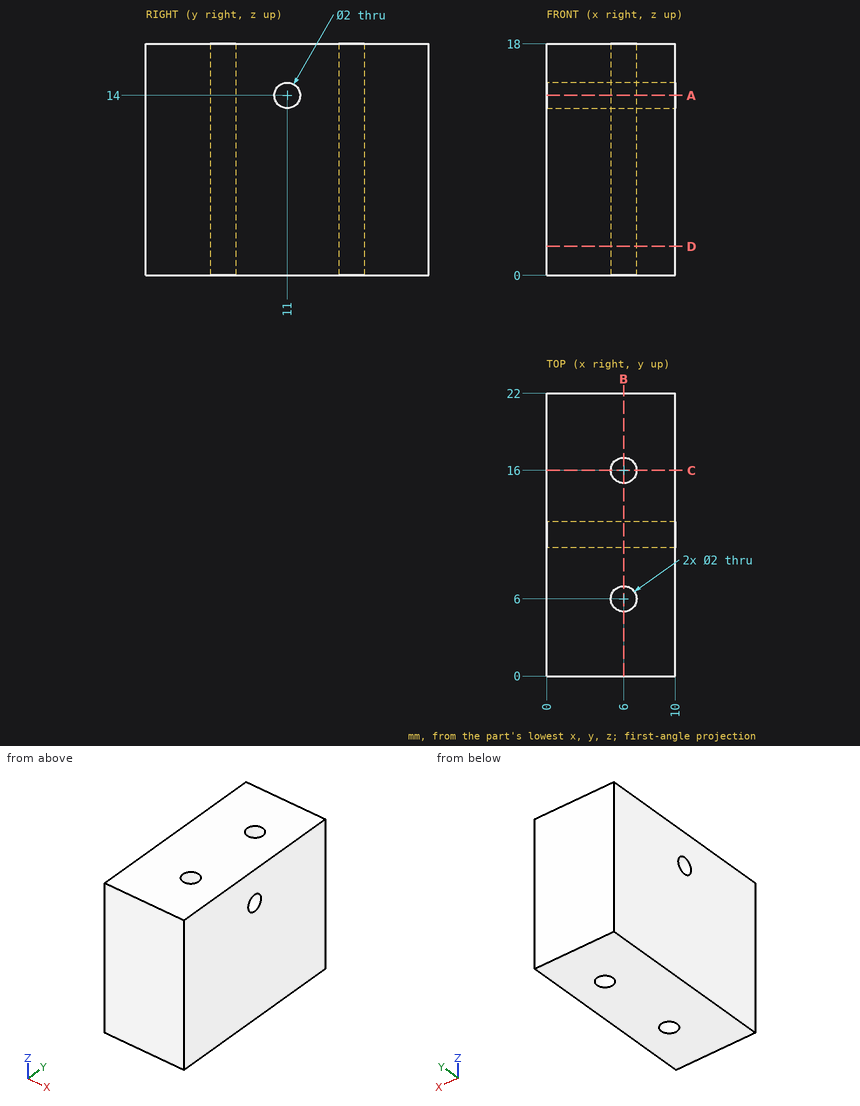
Input: dimensioned drawing with shaded views. Units: mm. Origin: part minimum x, y, z. Give positions to 0.01 mm unless a question says otherwise; leave off trailing zeros. Order: outer loops, then holes, each group sorted by start corner. A loop starts at its lowest first (then second) coordinate and runs counter-clockwise, first axis right, second up. Notation, with made-up numbers: (-33.5, -2.5) -> (-27.5, -2.5) arc R20 ccw to (-27.5, 21.5) -> close; hole circle Ø7 at (-19, -39.5). An arc over 180 degrees is marked (long way). Write item = value, one per line.
Item 1: Section query B-B (x = 6). Output: boundary loops of the cut face in (y, z), then the cut area to 3 significant figures.
Check result:
outline = (0, 0) -> (5, 0) -> (5, 18) -> (0, 18) -> close; (7, 0) -> (15, 0) -> (15, 18) -> (7, 18) -> close; (17, 0) -> (22, 0) -> (22, 18) -> (17, 18) -> close; hole circle Ø2 at (11, 14)
area = 321 mm²
Item 2: Ray query, probe 1 along Y at (x, z) = (6, 12); probe 2 along X at (y, z) = (6, 8); probe 3 along X at (y, z) = (6.5, 3). Return the intervals inside material, ascending.
Check result:
probe_1 = 0 to 5, 7 to 15, 17 to 22
probe_2 = 0 to 5, 7 to 10
probe_3 = 0 to 5.13, 6.87 to 10
Item 3: Section query C-C (y = 16). Output: boundary loops of the cut face in (x, z), then the cut area to 3 significant figures.
Check result:
outline = (0, 0) -> (5, 0) -> (5, 18) -> (0, 18) -> close; (7, 0) -> (10, 0) -> (10, 18) -> (7, 18) -> close
area = 144 mm²
Item 4: Contact query for a flat-ended pin moving along its axis: pin 1 (1.6 mm diameter, centred on x = 6, y = 16, fed in from -Z) (3 decimals). Output: stop coordinate, or through.
Check result:
pin_1 = through
Item 5: Section query A-A (z = 14). Output: boundary loops of the cut face in (x, y).
Check result:
outline = (0, 0) -> (10, 0) -> (10, 10) -> (0, 10) -> close; (0, 12) -> (10, 12) -> (10, 22) -> (0, 22) -> close; hole circle Ø2 at (6, 6); hole circle Ø2 at (6, 16)
Item 6: Section query D-D (z = 2.25). Output: boundary loops of the cut face in (x, y).
Check result:
outline = (0, 0) -> (10, 0) -> (10, 22) -> (0, 22) -> close; hole circle Ø2 at (6, 6); hole circle Ø2 at (6, 16)
